CAD build for the part. Positions are in the model's coordinates, mm. Face numbers are marked on the shaded views. A direction names the side the tool comes from. Round coordinates to 2 decimals unless told otherwise and drop trailing zeros. Write each loop counter-clockwise with the first axis right and the second up, starting at its lowest first coordinate (ties: lowest second). Pieces come first, ordered by that corner, then holes. Notation, with made-up numbers: (67, -18) - (74, -18) arc R19 cw to (74, 1) - close; hole circle Ø9 at (65.25, 38.5). An arc over 180 degrees is marked (long way). Answer in a Markdown table with one row per item.
```python
from build123d import *

# Parameters (mm, degrees)
F4_SIZE  = 0.381
F5_W     = 1.5875
F5_H     = 5.08
F6_DEPTH = 12.7


with BuildPart() as f1:
    # F0 (on Front) → F1 (revolve)
    with BuildSketch(Plane.XZ):
        Polygon((0, 53.975), (0, 0), (4.953, 0), (4.953, 38.1), (9.525, 38.1), (9.525, 44.45), (6.35, 44.45), (6.35, 53.975), align=None)
    revolve(axis=Axis((0, 0, 26.9875), (0, 0, 1)))

    # F2 (on Front) → F3 (revolve, cut)
    with BuildSketch(Plane.XZ):
        Polygon((0, -0.254), (4.064, -0.254), (4.064, 2.286), (2.814903, 3.175), (2.939943, 55.497955), (0, 55.50498), (0, 53.903468), (0, 51.516321), align=None)
    revolve(axis=Axis((0, 0, 26.824734), (0, 0, 1)), mode=Mode.SUBTRACT)

    # F4
    f4_edges = [f1.edges().sort_by_distance(p)[0] for p in [
        (-6.35, 0, 53.975),
    ]]
    chamfer(f4_edges, length=F4_SIZE)

    # F5 (on Front) → F6 (cut, symmetric)
    with BuildSketch(Plane.XZ):
        with Locations((6.33095, 49.2125)):
            Rectangle(F5_W, F5_H)
    extrude(amount=F6_DEPTH, both=True, mode=Mode.SUBTRACT)


solid = f1.part
```
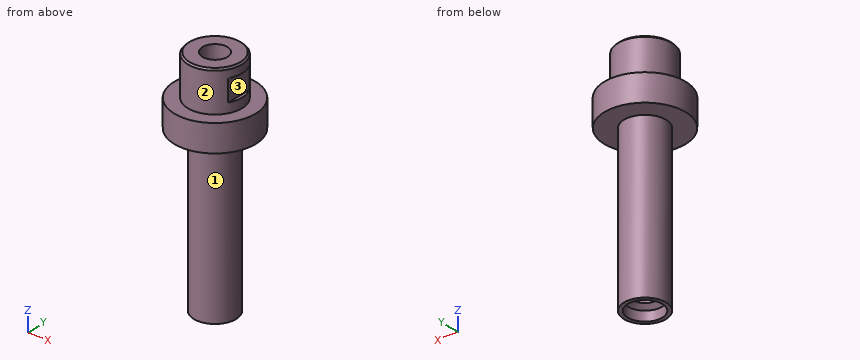
Q1. Saw through at D-D on z = 50. List the corners of the cut face in (x, y).
Computed:
| item | result |
|---|---|
| outline | (5.54, -3.11) - (5.54, 3.11) arc R6.35 ccw (long way) to start; hole circle Ø5.85 at (0, 0) |
Q2. Saw through at C-C on z = 19.5. List the corners of the cut face in (x, y).
Computed:
| item | result |
|---|---|
| outline | circle Ø9.91 at (0, 0); hole circle Ø5.71 at (0, 0) |
Q3. Flat gauge pins, fed straight in: pin 1 (1.5 mm diameter, centred on y = 1.5, z = 49, fed in from +X); pin 2 (10 mm diameter, centred on y = 1.5, z = 31, fed in from +X); pin 3 (6 mm diameter, centred on y = 4, z = 21.5, fed in from -X); pin 4 (0.7 mm diameter, centred on x = 6, y = 0.5, fed in from +Z) (3 decimals). Where does each tip first touch, or does it go through?
Computed:
| item | result |
|---|---|
| pin 1 | stops at x = 5.54 |
| pin 2 | stops at x = 4.95 |
| pin 3 | stops at x = -4.85 |
| pin 4 | stops at z = 53.975 |
Q4. Saw through at A-A on z = 33.5. List the corners of the cut face in (x, y), then the cut area to 3 significant figures.
Computed:
| item | result |
|---|---|
| outline | circle Ø9.91 at (0, 0); hole circle Ø5.77 at (0, 0) |
| area | 50.9 mm2 |
Q5. Drill centre lines: line 1 (Y direction, x = 0, z = 1.85); line 2 (Z direction, x = -6.5, y = -0.5); line 3 (X direction, y = -1.5, z = 31.5). Where is each one in solid material? Low to high.
Computed:
| item | result |
|---|---|
| line 1 | y = -4.95 to -4.06, 4.06 to 4.95 |
| line 2 | z = 38.1 to 44.45 |
| line 3 | x = -4.72 to -2.46, 2.46 to 4.72 |
Q6. Saw through at B-B on y = -7. List the corners of the cut face in (x, z).
Computed:
| item | result |
|---|---|
| outline | (-6.46, 38.1) - (6.46, 38.1) - (6.46, 44.45) - (-6.46, 44.45) - close |
Q7. 3-axis set-ups, long thin cutter, end or side, ignore diameter. For the marked faces 1, 2 and 3: which of +Z, -Z, +X, -X, +Y, -Y reach the whole face in a straight line?
Computed:
| item | result |
|---|---|
| face 1 | -Z |
| face 2 | +Z |
| face 3 | +X, +Y, -Y |
